CAD build for the part. Positions are in the model's coordinates, mm. A direction names the side the tool comes from. Coordinates: 2 decimals unless noted, no trailing zeros. Loops run counter-clockwise (first coordinate to the right, second up) from the corner with the lowest first, then second, coordinate; pieces in that order, holes last.
1) Which spindle directions (+Z, -Z, +X, -X, +Y, -Y) get a long thin tool onto all of the face, cutting with end or side? Do faces 4 (the flat face through (-4, -4.623, 2)), 5 (the flat face through (6, 0, 0)), 6 (the flat face through (-6, 0, 0)). Say none if no direction does.
2) Two-plate mould, pull along Z, no slides. Class faces 1 (the cylindrical face through (1.27, -1.48, 3.07)), 2 (the flat face through (0, -2, -10)), 3 (the cylindrical face through (7.46, -1.11, -0.14)): +Z half, -Z half, draft (parallel to the pull), parting line (faces both ways), or undercut.
3) Wall check: line 1 along Z through (x, y) = (0, -0.8); line 2 along Y through (x, z) = (-3, -7); line 3 along X through (y, z) = (-1.25, -2). Give the ranges that are in metal, low to high.
4) Pin check, flat tips, straight feed: pin 1 Ø1 at (y, z) = (-5, 6) entering from -X; pin 2 Ø5 at (y, z) = (-2.5, -0.5) entering from -X; pin 3 Ø1.4 at (x, y) = (4, -9.5) entering from -Z; pin 4 Ø0.5 at (y, z) = (1, -4.5) entering from -X. Stop position of each tip, or through.
5) Saw through at A-A, the plane x = 0. Write the cut outline in (y, z).
6) Saw through at C-C, the plane y = -8. Write the cut outline in (x, z).
7) Saw through at D-D, the plane y = -1. Write the cut outline in (x, z), and give its area (3 significant figures).
Autodesk Inventor part; units mm, degrees
ref_plane "YZ Plane" through (0, 0, 0) normal (1, 0, 0) x (0, 1, 0)
ref_plane "XZ Plane" through (0, 0, 0) normal (0, 1, 0) x (-1, 0, 0)
ref_plane "XY Plane" through (0, 0, 0) normal (0, 0, 1) x (1, 0, 0)
sketch "Sketch1" plane through (0, 0, 0) normal (0, 0, 1) x (1, 0, 0)
  line L0 (-4.8895, 1.7272) -> (4.8895, 1.7272)
  line L1 (4.8895, 1.7272) -> (4.8895, 0)
  line L2 (4.8895, 0) -> (7.4295, 0)
  line L3 (-4.8895, 1.7272) -> (-4.8895, 0)
  line L4 (-4.8895, 0) -> (-7.4295, 0)
  line L5 (0, 1.7272) -> (0, -4.6228) construction
  line L6 (-5.8161, -4.6228) -> (5.8161, -4.6228)
  arc A0 (5.8161, -4.6228) -> (7.4295, 0) centre (0, 0) ccw
  arc A1 (-7.4295, 0) -> (-5.8161, -4.6228) centre (0, 0) ccw
  dimension "d0" = 14.859
  dimension "d1" = 9.779
  dimension "d2" = 1.7272
  dimension "d3" = 6.35
extrude "Extrusion1" add sketch "Sketch1" along normal mid plane 20
sketch "Sketch2" plane through (-4.8895, 1.7272, 10) normal (0, 1, 0) x (1, 0, 0)
  point P0 (4.8895, 10)
  point P1 (4.8895, 10)
hole "Hole1" at (0, 1.7272, 0) direction (0, -1, 0) diameter 6.647 end through all
sketch "Sketch3" plane through (0, 0, 0) normal (0, 0, 1) x (1, 0, 0)
  line L0 (2.54, -11.4938) -> (4.321, -11.4938)
  arc A0 (4.321, -11.4938) -> (4.4305, -11.4115) centre (4.321, -11.3798) ccw
  line L1 (4.4305, -11.4115) -> (7.1364, -2.0663)
  line L2 (7.2459, -2.098) -> (4.54, -11.4432)
  arc A1 (4.321, -11.6078) -> (4.54, -11.4432) centre (4.321, -11.3798) ccw
  line L3 (4.321, -11.6078) -> (2.54, -11.6078)
  line L4 (2.54, -11.6078) -> (2.54, -11.4938)
  arc A2 (7.2459, -2.098) -> (7.5435, 0) centre (0, 0) ccw
  line L5 (7.4295, 0) -> (7.5435, 0)
  arc A3 (7.1364, -2.0663) -> (7.4295, 0) centre (0, 0) ccw
  line L6 (7.4295, 0) -> (4.8895, 0)
  line L7 (4.8895, 1.7272) -> (-4.8895, 1.7272)
  dimension "d16" = 0.114
  dimension "d17" = 0.114
  dimension "d18" = 2
  dimension "d20" = 13.335
  dimension "d21" = 2.54
extrude "Extrusion2" add sketch "Sketch3" along normal mid plane 20
sketch "Sketch4" plane through (7.1364, -2.0663, -10) normal (-0.9605462, 0.2781205, 0) x (0, 0, 1)
  line L0 (10, 0) -> (10, 0)
  line L1 (15, -5) -> (15, -10.4434)
  line L2 (15, -10.4434) -> (5, -10.4434)
  line L3 (5, -10.4434) -> (5, -5)
  line L4 (20, -10.4434) -> (0, -10.4434)
  arc A0 (15, -5) -> (10, 0) centre (10, -5) ccw
  arc A1 (10, 0) -> (5, -5) centre (10, -5) ccw
  line L5 (20, 0) -> (0, 0)
  point P0 (10, 0)
  point P1 (10, -10.4434)
  dimension "d24" = 10
  dimension "d25" = 5
extrude "Extrusion3" cut sketch "Sketch4" against normal through all
sketch "Sketch5" plane through (7.2459, -2.098, 10) normal (0.9605462, -0.2781205, 0) x (0, 0, -1)
  line L0 (5, -5) -> (15, -5)
  line L1 (15, -5) -> (15, -10.4434)
  line L2 (15, -10.4434) -> (5, -10.4434)
  line L3 (5, -10.4434) -> (5, -5)
  line L4 (0, -10.4434) -> (20, -10.4434)
  line L5 (15, -5) -> (15, -9.7291)
extrude "Extrusion4" cut sketch "Sketch5" against normal blind 3
fillet "Fillet1" radius 0.5 4 edges at (2.54, -11.5508, 10) (2.54, -11.5508, 5) (2.54, -11.5508, -5) (2.54, -11.5508, -10)
fillet "Fillet2" radius 0.125 6 edges at (4.8895, 1.7272, 0) (-4.8895, 1.7272, 0) (-7.4295, 0, 0) (5.8161, -4.6228, 0) (-5.8161, -4.6228, 0) (7.5435, 0, 0)
chamfer "Chamfer1" distance 0.625 angle 45 2 edges at (0, 1.7272, -3.3235) (0, -4.6228, -3.3235)
equation "\"d16\" = d17"
properties part number "NUT, SPRING, MK, M8" material "Steel, MS"
Data:
1. face 4: +Z, -Z, -X
1. face 5: +Z, -Z, +X, +Y
1. face 6: +Z, -Z, -X, +Y
2. face 1: undercut
2. face 2: -Z half
2. face 3: draft
3. line 1: z = -10 to -3.32, 3.32 to 10
3. line 2: y = -4.62 to 1.73
3. line 3: x = -7.32 to -2.65, 2.65 to 7.44
4. pin 1: stops at x = -5.91
4. pin 2: stops at x = -7.43
4. pin 3: passes through
4. pin 4: stops at x = -4.89
5. outline: (-4.62, -10) - (1.73, -10) - (1.73, -3.95) - (1.1, -3.32) - (-4, -3.32) - (-4.62, -3.95) - close; (-4.62, 3.95) - (-4, 3.32) - (1.1, 3.32) - (1.73, 3.95) - (1.73, 10) - (-4.62, 10) - close
6. outline: (5.42, -10) - (5.54, -10) - (5.54, -5) - (5.42, -5) - close; (5.42, 5) - (5.54, 5) - (5.54, 10) - (5.42, 10) - close
7. outline: (-7.36, -10) - (7.48, -10) - (7.48, 10) - (-7.36, 10) - close; hole circle Ø6.65 at (0, 0)
7. area: 262 mm2
